Can you work these out from the model? Positions are in its coordinate system, mm. A direction names the side the tool comes from. Round coordinates to 2 decimals unless told otherwise and drop trailing zeros. Loops run counter-clockwise (first coordinate to the right, second up) from the corner with the lowest first, then second, coordinate; pieces in that order, holes last. Notation, with made-up numbers: (23, -14) -> (47, -14) arc R11 cw to (47, -9) -> close; hole circle Ø10 at (3, 39.25). An arc over 180 degrees is marked (long way). Answer as a JSON object with one key per item and string values.
```python
from build123d import *

# Parameters (mm, degrees)
F0_W       = 38.89502
F0_H       = 121.158
F1_DEPTH   = 38.1
F2_SIZE    = 10.922
F3_R       = 12.7
F4_SIZE2   = 5.08
F4_SIZE    = 38.1
F4_2_SIZE2 = 5.08
F4_2_SIZE  = 38.1
F5_R       = 12.3825
F6_R       = 5.08
F6_R_2     = 3.556
F7_DEPTH   = 12.7
F8_DEPTH   = 38.101


with BuildPart() as f1:
    # F0 (on Front) → F1 (new body)
    with BuildSketch(Plane.XZ):
        with Locations((0, -9.779)):
            Rectangle(F0_W, F0_H)
    extrude(amount=-F1_DEPTH)

    # F2
    f2_edges = [f1.edges().sort_by_distance(p)[0] for p in [
        (19.44751, 19.05, 50.8),
        (-19.44751, 19.05, 50.8),
    ]]
    chamfer(f2_edges, length=F2_SIZE)

    # F3
    f3_edges = [f1.edges().sort_by_distance(p)[0] for p in [
        (19.44751, 19.05, 39.878),
        (-19.44751, 19.05, 39.878),
    ]]
    fillet(f3_edges, radius=F3_R)

    # F4
    f4_edges = [f1.edges().sort_by_distance(p)[0] for p in [
        (-19.44751, 19.05, -70.358),
    ]]
    f4_side = f1.faces().sort_by_distance((-19.44751, 19.05, -17.870256))[0]
    chamfer(f4_edges, length=F4_SIZE, length2=F4_SIZE2, reference=f4_side)

    # F4#2
    f4_2_edges = [f1.edges().sort_by_distance(p)[0] for p in [
        (19.44751, 19.05, -70.358),
    ]]
    f4_2_side = f1.faces().sort_by_distance((19.44751, 19.05, -17.870256))[0]
    chamfer(f4_2_edges, length=F4_2_SIZE, length2=F4_2_SIZE2, reference=f4_2_side)

    # F5
    f5_edges = [f1.edges().sort_by_distance(p)[0] for p in [
        (14.36751, 19.05, -70.358),
        (-14.36751, 19.05, -70.358),
    ]]
    fillet(f5_edges, radius=F5_R)

    # F6 (on face) → F7 (cut)
    with BuildSketch(Plane(origin=(0, 38.1, 0), x_dir=(-1, 0, 0), z_dir=(0, 1, 0))):
        with Locations((0, -39.878)):
            Circle(F6_R)
        with Locations((0, -39.878)):
            Circle(F6_R_2, mode=Mode.SUBTRACT)
        with Locations((0, -10.16)):
            Circle(F6_R)
        with Locations((0, -10.16)):
            Circle(F6_R_2, mode=Mode.SUBTRACT)
        with Locations((0, 20.32)):
            Circle(F6_R)
        with Locations((0, 20.32)):
            Circle(F6_R_2, mode=Mode.SUBTRACT)
    extrude(amount=-F7_DEPTH, mode=Mode.SUBTRACT)

    # F6 (on face) → F8 (cut, through all)
    with BuildSketch(Plane(origin=(0, 38.1, 0), x_dir=(-1, 0, 0), z_dir=(0, 1, 0))):
        with Locations((0, 20.32)):
            Circle(F6_R_2)
        with Locations((0, -10.16)):
            Circle(F6_R_2)
        with Locations((0, -39.878)):
            Circle(F6_R_2)
    extrude(amount=-F8_DEPTH, mode=Mode.SUBTRACT)


solid = f1.part
```
Q1. I want a section at D-D, the plane x = 14. Write out the boundary of the cut face in (y, z).
Determined:
{"outline": "(0, -64.58) -> (38.1, -64.58) -> (38.1, 45.33) -> (0, 45.33) -> close"}
Q2. I want a section at B-B, the plane z = -10.16. Write out the boundary of the cut face in (x, y), then the cut area to 3 significant figures.
Determined:
{"outline": "(-19.45, 0) -> (-3.56, 0) -> (-3.56, 25.4) -> (-5.08, 25.4) -> (-5.08, 38.1) -> (-19.45, 38.1) -> close; (3.56, 0) -> (19.45, 0) -> (19.45, 38.1) -> (5.08, 38.1) -> (5.08, 25.4) -> (3.56, 25.4) -> close", "area": "1,170 mm²"}
Q3. I want a section at C-C, the plane y = 19. Write out the boundary of the cut face in (x, z) (1 decimal), then the cut area to 3 significant figures.
Determined:
{"outline": "(-19.4, -32.3) -> (-15.8, -59.6) arc R12.4 ccw to (-3.5, -70.4) -> (3.5, -70.4) arc R12.4 ccw to (15.8, -59.6) -> (19.4, -32.3) -> (19.4, 34.6) arc R12.7 ccw to (15.7, 43.6) -> (8.5, 50.8) -> (-8.5, 50.8) -> (-15.7, 43.6) arc R12.7 ccw to (-19.4, 34.6) -> close; hole circle Ø7.1 at (0, -39.9); hole circle Ø7.1 at (0, -10.2); hole circle Ø7.1 at (0, 20.3)", "area": "4,230 mm²"}
Q4. I'm going to push flat-ended pins straight in: pin 1 (1.5 mm diameter, centred on y = 22, z = -45, fed in from -X); pin 2 (3 mm diameter, centred on x = -1, z = -37.5, fed in from +Y); pin 3 (5 mm diameter, centred on x = -12.5, y = 14.5, fed in from -Z). Where does each tip first touch, or does it pass through?
Determined:
{"pin 1": "x = -17.85", "pin 2": "y = 25.4", "pin 3": "z = -68.53"}
Q5. If I drill on L1, parallel to Z at x = 0, y = 30; L2, parallel to Z at x = 0, y = 5.75; L3, parallel to X at y = 32, z = -10, over which ranges is the centre line in solid material (lowest first)? Write a range as [from, to].
Determined:
{"L1": "[-70.36, -44.96], [-34.8, -15.24], [-5.08, 15.24], [25.4, 50.8]", "L2": "[-70.36, -43.43], [-36.32, -13.72], [-6.6, 16.76], [23.88, 50.8]", "L3": "[-19.45, -5.08], [5.08, 19.45]"}
Q6. I want a section at A-A, the plane x = 0. Write out the boundary of the cut face in (y, z).
Determined:
{"outline": "(0, -70.36) -> (38.1, -70.36) -> (38.1, -44.96) -> (25.4, -44.96) -> (25.4, -43.43) -> (0, -43.43) -> close; (0, -36.32) -> (25.4, -36.32) -> (25.4, -34.8) -> (38.1, -34.8) -> (38.1, -15.24) -> (25.4, -15.24) -> (25.4, -13.72) -> (0, -13.72) -> close; (0, -6.6) -> (25.4, -6.6) -> (25.4, -5.08) -> (38.1, -5.08) -> (38.1, 15.24) -> (25.4, 15.24) -> (25.4, 16.76) -> (0, 16.76) -> close; (0, 23.88) -> (25.4, 23.88) -> (25.4, 25.4) -> (38.1, 25.4) -> (38.1, 50.8) -> (0, 50.8) -> close"}
Q7. On a 3-axis mill with a long thin cutter (end or side, diameter ignored), from which of +Z, -Z, +X, -X, +Y, -Y can I reach the whole of each face in a straight line? I mean faces 4 (the flat face through (-1, 25.4, -36)), 5 (the flat face through (-17.6, 18.8, -46.1)). Say none if no direction works.
Determined:
{"face 4": "+Y", "face 5": "-Z, -X, +Y, -Y"}
Q8. We'd pull the mould along Z, two halves only. Please class faces 1 (the flat face through (17.6, 18.8, -46.1)), 2 (the cylindrical face through (0.463, 12.878, 23.846)), 3 (the flat face through (0, 19, 50.8)): pulls with the +Z half, pulls with the -Z half, needs draft (parallel to the pull), parting line crosses it, or undercut.
Determined:
{"face 1": "pulls with the -Z half", "face 2": "undercut", "face 3": "pulls with the +Z half"}
